Can you work these out from the model? Positions are in its coordinate system, mm. Round coordinates to 2 decimals unless told otherwise and drop trailing zeros. Order: outer loops, then holes, each group sorted by start corner. A loop starts at its lowest first (then second) coordinate and runs counter-clockwise, first axis right, second up. Notation, with made-up numbers: M 33.5,76 L 71.5,76 A16 cw 71.5,88 Z; hole C -32.5,-28.5 d5. An arc over 180 degrees is marked long. Answer as a JSON object with one key per item and string values. Group by question number.
```python
from build123d import *

# Parameters (mm, degrees)
BOSS_EXTRU_1_DEPTH = 5


with BuildPart() as part:
    # Esquisse1 → Boss.-Extru.1 (new body)
    with BuildSketch(Plane(origin=(0, 0, 0), x_dir=(1, 0, 0), z_dir=(0, 1, 0))):
        with BuildLine():
            Line((-42.5, 40), (1.075699519, 40))
            Line((1.075699519, 40), (7.256174968, 34.16461456))
            ThreePointArc((7.256174968, 34.16461456), (8.582181318, 6.457704827), (36.319524552, 6.724031969))
            Line((36.319524552, 6.724031969), (42.5, 0.88864653))
            Line((42.5, 0.88864653), (42.5, -40))
            Line((42.5, -40), (-42.5, -40))
            Line((-42.5, -40), (-42.5, 40))
        make_face()
    extrude(amount=BOSS_EXTRU_1_DEPTH)


solid = part.part
```
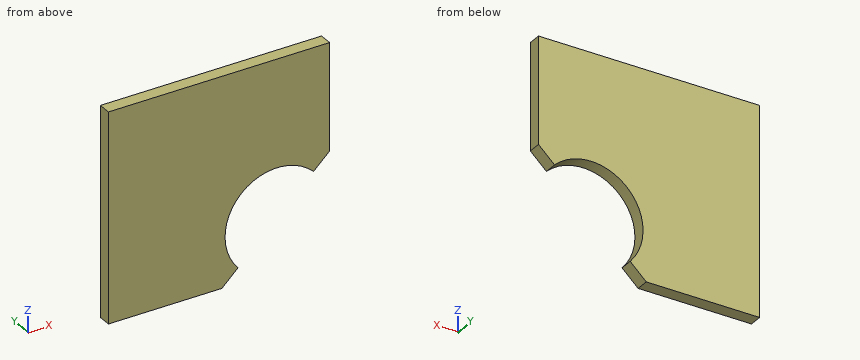
1) If we section it at B-B on z = -21: Write out the boundary of the cut face in (x, y), plus the area to 3 significant figures.
2) If we section it at C-C on x = 31: Write out the boundary of the cut face in (y, z), plus the area to 3 significant figures.
3) If we section it at A-A on y = 2: Write out the boundary of the cut face in (x, z), plus the area to 3 significant figures.
4) I need wall thicknesses on line 1 along Z through (x, y) = (21.5, 2.95); line 2 along Z through (x, y) = (6.5, 2.55); line 3 along X through (y, z) = (1.5, -32). Which ranges of each line are inside material? Lowest first, please.
Findings:
{
 "1": {"outline": "M -42.5,0 L 2.31,0 L 2.31,5 L -42.5,5 Z", "area": "224 mm^2"},
 "2": {"outline": "M 0,-2.99 L 5,-2.99 L 5,40 L 0,40 Z", "area": "215 mm^2"},
 "3": {"outline": "M -42.5,-40 L 1.08,-40 L 7.26,-34.16 A20 cw 36.32,-6.72 L 42.5,-0.89 L 42.5,40 L -42.5,40 Z", "area": "5,390 mm^2"},
 "4": {"line 1": "z = -1.02 to 40", "line 2": "z = -34.88 to -33.25, -8.75 to 40", "line 3": "x = -42.5 to 5.61"}
}
